from build123d import *

# Parameters (mm, degrees)
F0_R        = 15
F1_DEPTH    = 6.5
F2_R        = 5
F3_R        = 10
F3_R_2      = 7.5
F4_DEPTH    = 25
F5_SIZE     = 1
F6_SIZE     = 1
F7_T2_ANGLE = 180
F7_T4_ANGLE = 180


# Not quite as in the source:
# - a fillet or chamfer that OpenCascade refuses, or shapes differently, is made with other operations: its cross-section is extruded or revolved along the edge and cut away or added


with BuildPart() as f1:
    # F0 (on Front) → F1 (new body)
    with BuildSketch(Plane.XZ):
        Circle(F0_R)
    extrude(amount=-F1_DEPTH)

    # F2
    f2_edges = [f1.edges().sort_by_distance(p)[0] for p in [
        (-15, 6.5, 0),
    ]]
    fillet(f2_edges, radius=F2_R)

    # F3 (on face) → F4 (join)
    with BuildSketch(Plane(origin=(0, 6.5, 0), x_dir=(-1, 0, 0), z_dir=(0, 1, 0))):
        Circle(F3_R)
        Circle(F3_R_2, mode=Mode.SUBTRACT)
    extrude(amount=F4_DEPTH)

    # F5
    f5_edges = [f1.edges().sort_by_distance(p)[0] for p in [
        (7.5, 31.5, 0),
    ]]
    chamfer(f5_edges, length=F5_SIZE)

    # F6
    f6_edges = [f1.edges().sort_by_distance(p)[0] for p in [
        (10, 31.5, 0),
    ]]
    chamfer(f6_edges, length=F6_SIZE)

    # F7: chamfer of 5 on 2 edges, made by hand

    # F7_s1 → F7_t2 (revolve)
    with BuildSketch(Plane.XY):
        with BuildLine():
            Line((10, 10.1602540378), (12.5, 5.8301270189))
            ThreePointArc((12.5, 5.8301270189), (11.3657058128, 6.3098698146), (10, 6.5))
            Line((10, 6.5), (10, 10.1602540378))
        make_face()
    revolve(axis=Axis((0, 6.5, 0), (0, -1, 0)), revolution_arc=F7_T2_ANGLE)

    # F7_s3 → F7_t4 (revolve)
    with BuildSketch(Plane.XY):
        with BuildLine():
            Line((-10, 10.1602540378), (-12.5, 5.8301270189))
            ThreePointArc((-12.5, 5.8301270189), (-11.3657058128, 6.3098698146), (-10, 6.5))
            Line((-10, 6.5), (-10, 10.1602540378))
        make_face()
    revolve(axis=Axis((0, 6.5, 0), (0, -1, 0)), revolution_arc=F7_T4_ANGLE)


solid = f1.part
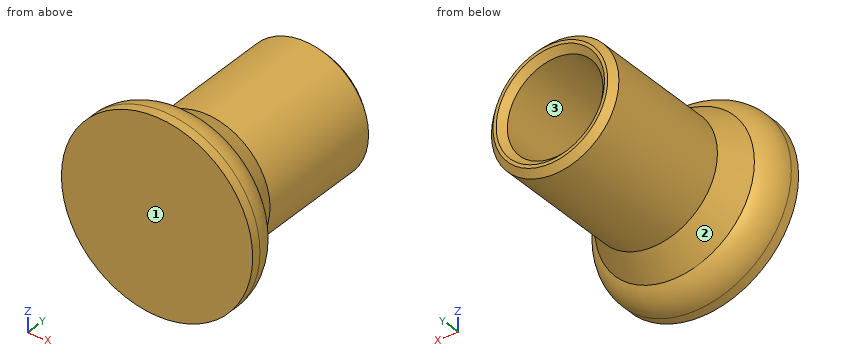
CAD build for the part. Positions are in the model's coordinates, mm. Face numbers are marked on the shaded views. Coordinates: 2 decimals unless noted, no trailing zeros. Loops run counter-clockwise (first coordinate to the right, second up) from the corner with the lowest first, then second, coordinate; pieces in that order, holes last. Notation, with made-up numbers: (40.25, 80) - (82.25, 80) arc R6 ccw to (82.25, 86) - close; hole circle Ø1 at (51.5, -5.75). An arc over 180 degrees is marked (long way). Use one line per item in the form item = value. Start each with the question number.
1) Band-saw the part on B-B (x = 0). Give the cut face in (y, z).
2) Drill centre lines: L1, parallel to Z at x = 0, y = 12.75; L2, parallel to Z at x = 4.5, y = 14; L3, parallel to X at y = 20, z = -3. Where is each one in solid material? Low to high. Write a range as from..to.
3) Band-saw the part on D-D (y = 5). Give the cut face in (x, z).
4) Band-saw the part on A-A (y = 13.5). Give the cut face in (x, z).
5) Flat gauge pins, fed straight in: pin 1 (10 mm diameter, centred on x = 12, y = 10, fed in from -Z); pin 2 (4 mm diameter, centred on y = 8, z = -2, fed in from -X); pin 3 (12 mm diameter, centred on x = 0.5, y = 18.5, fed in from +Z). Where does each tip first touch, or does it go through?
6) Band-saw the part on C-C (z = 0). Give the cut face in (x, y), and give its area (3 significant figures).
7) Two-plate mould, pull along Z, no slides. Class the marked faces 1, 2 and 3: +Z half, -Z half, draft (parallel to the pull), parting line (faces both ways), or undercut.
Check values:
q1.outline = (0, -15) - (1.5, -15) arc R5 ccw to (5.83, -12.5) - (10.16, -10) - (30.5, -10) - (31.5, -9) - (31.5, -8.5) - (30.5, -7.5) - (6.5, -7.5) - (6.5, 7.5) - (30.5, 7.5) - (31.5, 8.5) - (31.5, 9) - (30.5, 10) - (10.16, 10) - (5.83, 12.5) arc R5 ccw to (1.5, 15) - (0, 15) - close
q2.L1 = -10..-7.5, 7.5..10
q2.L2 = -8.93..-6, 6..8.93
q2.L3 = -9.54..-6.87, 6.87..9.54
q3.outline = circle Ø27.14 at (0, 0)
q4.outline = circle Ø20 at (0, 0); hole circle Ø15 at (0, 0)
q5.pin_1 = -8.72
q5.pin_2 = -12.27
q5.pin_3 = 10
q6.outline = (-15, 0) - (15, 0) - (15, 1.5) arc R5 ccw to (12.5, 5.83) - (10, 10.16) - (10, 30.5) - (9, 31.5) - (8.5, 31.5) - (7.5, 30.5) - (7.5, 6.5) - (-7.5, 6.5) - (-7.5, 30.5) - (-8.5, 31.5) - (-9, 31.5) - (-10, 30.5) - (-10, 10.16) - (-12.5, 5.83) arc R5 ccw to (-15, 1.5) - close
q6.area = 316 mm2
q7.face_1 = draft
q7.face_2 = parting line
q7.face_3 = undercut
